The model under review builds one solid part; all positions refer to its coordinate system, in mm. A direction names the side the tool comes from. Coordinates: 2 decimals unless noted, no trailing zeros. Order: outer loops, then holes, each group sorted by start corner. A loop starts at its lowest first (then second) coordinate and runs counter-clockwise, first axis right, second up. Notation, with made-up numbers: M 29,26.5 L 58,26.5 A11 cw 58,47.5 Z; hole C 56,74 d1. An arc over 180 degrees is marked long. Answer in a Markdown table with one row per item.
from build123d import *

# Parameters (mm, degrees)
F3_DEPTH   = 3
F4_R       = 2.5
F5_DEPTH   = 1.5
F6_R       = 3
F7_DEPTH   = 14.5
F8_SIZE2   = 0.2886751346
F8_SIZE    = 0.5
F8_2_SIZE2 = 0.288665
F8_2_SIZE  = 0.49999


# Not quite as in the source:
# - a fillet or chamfer is up to 0.001 mm smaller than in the source, because OpenCascade refuses the exact size


with BuildPart() as f1:
    # F0 (on Front) → F1 (revolve)
    with BuildSketch(Plane.XZ):
        Polygon((0, 2.4), (0, 0), (0.9, 0), (2.2856406461, 2.4), align=None)
    revolve(axis=Axis((-0.6, 0, 1.2), (0, 0, 1)))

    # F2 (on face) → F3 (join)
    with BuildSketch(Plane.XY.offset(2.4)):
        Polygon((2.9073034694, 2.0080228353), (-0.5853470521, 4.0414253209), (-4.0926505214, 2.0334024856), (-4.1073034694, -2.0080228353), (-0.6146529479, -4.0414253209), (2.8926505214, -2.0334024856), align=None)
    extrude(amount=F3_DEPTH)

    # F4 (on face) → F5 (join)
    with BuildSketch(Plane.XY.offset(5.4)):
        with Locations((-0.6, 0)):
            Circle(F4_R)
    extrude(amount=F5_DEPTH)

    # F6 (on face) → F7 (join)
    with BuildSketch(Plane.XY.offset(6.9)):
        with Locations((-0.6, 0)):
            Circle(F6_R)
    extrude(amount=F7_DEPTH)

    # F8
    f8_edges = [f1.edges().sort_by_distance(p)[0] for p in [
        (-3.6, 0, 21.4),
    ]]
    f8_side = f1.faces().sort_by_distance((-0.6, 0, 21.4))[0]
    chamfer(f8_edges, length=F8_SIZE, length2=F8_SIZE2, reference=f8_side)

    # F8#2 (size 0.5 and 0.2886751346 in the source; OpenCascade refuses exactly that, so slightly less here)
    f8_2_edges = [f1.edges().sort_by_distance(p)[0] for p in [
        (-3.6, 0, 6.9),
    ]]
    f8_2_side = f1.faces().sort_by_distance((-3.515147, 0, 6.9))[0]
    chamfer(f8_2_edges, length=F8_2_SIZE, length2=F8_2_SIZE2, reference=f8_2_side)


solid = f1.part
(1) To check wall thickness, follow line 1 (Z direction, x = -0.5, y = 0.25); line 2 (Z direction, x = -2, y = 3); line 3 (Y direction, x = 2, z = 13.5). State the ranges of each line that lie inside material, in increasing order. Write a range as [from, to].
Report:
| item | result |
|---|---|
| line 1 | [2.4, 21.4] |
| line 2 | [2.4, 5.4] |
| line 3 | [-1.5, 1.5] |
(2) Insertion check: P1, Ø1, axis at y = 1.5, z = 19, coming from the -X side; P2, Ø1, axis at x = -2, z = 3, coming from the +Y side; P3, Ø2, axis at x = -3, z = 18.5, coming from the -Y side. Each pin has a flat end and moves straight along its axis. Give the tip position at first contact, or say it passes through.
Report:
| item | result |
|---|---|
| P1 | x = -3.43 |
| P2 | y = 3.52 |
| P3 | y = -2.65 |
(3) Machinability: for faces 1 (the flat face through (-1, 0, 2.4)), 2 (the flat face through (-1, 0, 21.4)), 3 (the cylindrical face through (-1.14, -2.44, 6.14)), 4 (the flat face through (-1, -1, 0)), 5 (the cylindrical face through (-3.6, 0.1, 14.1)), which of the approach directions +Z, -Z, +X, -X, +Y, -Y give a long, thin tool a straight path to every point of the face, cutting with its end or side? Answer none if there is none.
Report:
| item | result |
|---|---|
| face 1 | -Z |
| face 2 | +Z, +X, -X, +Y, -Y |
| face 3 | none |
| face 4 | -Z, +X, -X, +Y, -Y |
| face 5 | +Z |
(4) Take a section at A-A (z = 4). Write out the cut boundary in (x, y), then the cut area to 3 significant figures.
Report:
| item | result |
|---|---|
| outline | M -4.11,-2.01 L -0.61,-4.04 L 2.89,-2.03 L 2.91,2.01 L -0.59,4.04 L -4.09,2.03 Z |
| area | 42.4 mm^2 |
(5) Take a section at C-C (z = 12). Write out the cut boundary in (x, y).
Report:
| item | result |
|---|---|
| outline | C -0.6,0 d6 |
(6) The part is to be moulded in two halves that separate along Y. For faces 6 (the flat face through (2, 2, 2.4)), 7 (the cylindrical face through (-1.2, 0, 1.2)), 8 (the flat face through (-2.4, -3, 3.9)), say which applies: +Y half, -Y half, draft (parallel to the pull), parting line (faces both ways), or undercut.
Report:
| item | result |
|---|---|
| face 6 | draft |
| face 7 | undercut |
| face 8 | -Y half |
